Geometry check sheet. Reference: the model listing, model coordinates, mm. Give positions to 0.01 mm unless a question says otherwise; leave off trailing zeros. Loops run counter-clockwise (first coordinate to the right, second up) from the corner with the lowest first, then second, coordinate; pieces in that order, holes last. Notation, with made-up numbers: (75.5, -10) -> (83.5, -10) arc R31 ccw to (83.5, 15) -> close; hole circle Ø9 at (86, 20). An arc over 180 degrees is marked (long way). One line per item, written item: value. Start each with the question number.
(1) Sectioned sample at A-A, the plane x = -8.5. Record the cut outline in (y, z), then the cut area to 3 significant figures.
(2) Gauge pin test, flat end, axial feed: pin 1 Ø2.5 at (x, z) = (-23.5, -48) entering from -Y. Record the tip position at first contact, or that the pin passes through.
(3) Sectioned sample at B-B, the plane y = 2. State how many separate pieces and enclosed holes the cut face has, then the cut area to 3 significant figures.
(4) Scan lines: line 1 along Z through (x, y) = (23, 3.1); line 2 along X through (y, z) = (3.2, 119); line 3 along Z through (x, y) = (-4, 2). Record each from-to range of solid material in increasing order. Write a range as from..to.
from build123d import *

# Parameters (mm, degrees)
SKETCH2_W           = 360
SKETCH2_H           = 250
SKETCH2_R           = 1.75
SKETCH2_R_2         = 1.5
SKETCH2_W_2         = 25
SKETCH2_H_2         = 25
BOSS_EXTRUDE1_DEPTH = 5
FILLET1_R           = 5


with BuildPart() as part:
    # Sketch2 → Boss-Extrude1 (new body)
    with BuildSketch(Plane(origin=(0, 0, 0), x_dir=(1, 0, 0), z_dir=(0, 1, 0))):
        Rectangle(SKETCH2_W, SKETCH2_H)
        with Locations(Location((-172.5, 95, 0), (0, 0, 270))):
            Circle(SKETCH2_R, mode=Mode.SUBTRACT)
        with Locations(Location((-172.5, 119, 0), (0, 0, 270))):
            Circle(SKETCH2_R, mode=Mode.SUBTRACT)
        with Locations(Location((-172.5, 71, 0), (0, 0, 270))):
            Circle(SKETCH2_R, mode=Mode.SUBTRACT)
        with Locations(Location((-115.5, 119, 0), (0, 0, 90))):
            Circle(SKETCH2_R, mode=Mode.SUBTRACT)
        with Locations(Location((-115.5, 95, 0), (0, 0, 90))):
            Circle(SKETCH2_R, mode=Mode.SUBTRACT)
        with Locations(Location((-115.5, 71, 0), (0, 0, 90))):
            Circle(SKETCH2_R, mode=Mode.SUBTRACT)
        with Locations(Location((172.5, 71, 0), (0, 0, 90))):
            Circle(SKETCH2_R, mode=Mode.SUBTRACT)
        with Locations(Location((172.5, 95, 0), (0, 0, 90))):
            Circle(SKETCH2_R, mode=Mode.SUBTRACT)
        with Locations(Location((172.5, 119, 0), (0, 0, 90))):
            Circle(SKETCH2_R, mode=Mode.SUBTRACT)
        with Locations(Location((115.5, 119, 0), (0, 0, 270))):
            Circle(SKETCH2_R, mode=Mode.SUBTRACT)
        with Locations(Location((115.5, 95, 0), (0, 0, 270))):
            Circle(SKETCH2_R, mode=Mode.SUBTRACT)
        with Locations(Location((115.5, 71, 0), (0, 0, 270))):
            Circle(SKETCH2_R, mode=Mode.SUBTRACT)
        with Locations(Location((-172.5, -119, 0), (0, 0, 90))):
            Circle(SKETCH2_R, mode=Mode.SUBTRACT)
        with Locations(Location((-172.5, -95, 0), (0, 0, 90))):
            Circle(SKETCH2_R, mode=Mode.SUBTRACT)
        with Locations(Location((-172.5, -71, 0), (0, 0, 90))):
            Circle(SKETCH2_R, mode=Mode.SUBTRACT)
        with Locations(Location((-115.5, -119, 0), (0, 0, 270))):
            Circle(SKETCH2_R, mode=Mode.SUBTRACT)
        with Locations(Location((-115.5, -95, 0), (0, 0, 270))):
            Circle(SKETCH2_R, mode=Mode.SUBTRACT)
        with Locations(Location((-115.5, -71, 0), (0, 0, 270))):
            Circle(SKETCH2_R, mode=Mode.SUBTRACT)
        with Locations(Location((115.5, -71, 0), (0, 0, 90))):
            Circle(SKETCH2_R, mode=Mode.SUBTRACT)
        with Locations(Location((115.5, -95, 0), (0, 0, 90))):
            Circle(SKETCH2_R, mode=Mode.SUBTRACT)
        with Locations(Location((115.5, -119, 0), (0, 0, 90))):
            Circle(SKETCH2_R, mode=Mode.SUBTRACT)
        with Locations(Location((172.5, -119, 0), (0, 0, 270))):
            Circle(SKETCH2_R, mode=Mode.SUBTRACT)
        with Locations(Location((172.5, -95, 0), (0, 0, 270))):
            Circle(SKETCH2_R, mode=Mode.SUBTRACT)
        with Locations(Location((172.5, -71, 0), (0, 0, 270))):
            Circle(SKETCH2_R, mode=Mode.SUBTRACT)
        with Locations(Location((-23.5, 101, 0), (0, 0, 270))):
            Circle(SKETCH2_R_2, mode=Mode.SUBTRACT)
        with Locations(Location((-23.5, -101, 0), (0, 0, 90))):
            Circle(SKETCH2_R_2, mode=Mode.SUBTRACT)
        with Locations(Location((-23.5, 0, 0), (0, 0, 270))):
            Circle(SKETCH2_R_2, mode=Mode.SUBTRACT)
        with Locations(Location((-23.5, 48, 0), (0, 0, 270))):
            Circle(SKETCH2_R_2, mode=Mode.SUBTRACT)
        with Locations(Location((-23.5, -48, 0), (0, 0, 270))):
            Circle(SKETCH2_R_2, mode=Mode.SUBTRACT)
        with Locations(Location((23.5, 101, 0), (0, 0, 90))):
            Circle(SKETCH2_R_2, mode=Mode.SUBTRACT)
        with Locations(Location((23.5, 48, 0), (0, 0, 90))):
            Circle(SKETCH2_R_2, mode=Mode.SUBTRACT)
        with Locations(Location((23.5, 0, 0), (0, 0, 90))):
            Circle(SKETCH2_R_2, mode=Mode.SUBTRACT)
        with Locations(Location((23.5, -48, 0), (0, 0, 90))):
            Circle(SKETCH2_R_2, mode=Mode.SUBTRACT)
        with Locations(Location((23.5, -101, 0), (0, 0, 270))):
            Circle(SKETCH2_R_2, mode=Mode.SUBTRACT)
        with Locations((0, 75)):
            Rectangle(SKETCH2_W_2, SKETCH2_H_2, mode=Mode.SUBTRACT)
        with Locations((0, -50)):
            Rectangle(SKETCH2_W_2, SKETCH2_H_2, mode=Mode.SUBTRACT)
    extrude(amount=BOSS_EXTRUDE1_DEPTH)

    # Fillet1
    fillet1_edges = [part.edges().sort_by_distance(p)[0] for p in [
        (-180, 2.5, -125),
        (180, 2.5, -125),
        (180, 2.5, 125),
        (-180, 2.5, 125),
    ]]
    fillet(fillet1_edges, radius=FILLET1_R)


solid = part.part
Calculated:
1. outline: (0, -125) -> (5, -125) -> (5, -87.5) -> (0, -87.5) -> close; (0, -62.5) -> (5, -62.5) -> (5, 37.5) -> (0, 37.5) -> close; (0, 62.5) -> (5, 62.5) -> (5, 125) -> (0, 125) -> close
1. area: 1,000 mm2
2. pin 1: passes through
3. separate pieces: 1
3. enclosed holes: 36
3. area: 88,400 mm2
4. line 1: z = -125..-102.41, -99.59..-49.41, -46.59..-1.41, 1.41..46.59, 49.41..99.59, 102.41..125
4. line 2: x = -180..-174.25, -170.75..-117.25, -113.75..113.75, 117.25..170.75, 174.25..180
4. line 3: z = -125..-87.5, -62.5..37.5, 62.5..125
